Here's how the part is built. I have some questions about the finished solid (model axes, mm). A direction names the side the tool comes from. Coordinates: 2 decimals unless noted, no trailing zeros. Write each loop counter-clockwise with the first axis right and the second up, starting at its lowest first coordinate (ties: lowest second). Pieces come first, ordered by that corner, then holes.
Item 1: I want a section at C-C (z = -1). Please give me the cut outline in (x, y), and give its area (3 significant figures).
Item 2: For faces 1 (the face through (18, 441.047, -4)), 2 (the face through (-6.469, 481, 3)), 3 (the face through (8, 482, 9.934)), 4 (the face through (13.531, 483, 5)), which set-ups out of +Z, -Z, +X, -X, +Y, -Y let a thin tool reach every point of the face, with its end or its side?
Item 3: I want a section at A-A (y = 483). Please give me the cut outline in (x, z).
Item 4: I want a section at D-D (x = -2.5). Please give me the cut outline in (y, z), and give its area (3 significant figures).
Item 5: I'm going to push flat-ended pins straight in: P1, Ø3, axis at x = -3.5, z = 18, coming from the +Y side; P2, Ø2.5, axis at x = -21, z = -3, coming from the +Y side; P3, Ø6, axis at y = 487.55, z = 4.93, coming from the +X side. Where does each tip first touch, or does it pass through?
Item 6: I want a section at B-B (x = -12). Please give me the cut outline in (y, z), and give its area (3 significant figures).
Item 7: If we mould it in two halves opening along Y, with no side actions, what happens to faces 5 (the face through (-8, 469.547, -1)), 6 (the face through (-12, 482, -0.066)), 7 (the face through (-2, 412.547, 29))? For each: pulls with the +Y half, pulls with the -Y half, needs draft (parallel to the pull), parting line crosses it, or undercut.
Item 8: Please list where these lines run through material, in increasing order: line 1 (Y direction, x = -6, z = 4); line 2 (X direction, y = 440.5, z = 3.5); line 3 (X direction, y = 427, z = 23).
from build123d import *

# Parameters (mm, degrees)
SKETCH1_W            = 50
SKETCH1_H            = 40
BOSS_EXTRUDE1_DEPTH  = 10
SKETCH5_W            = 6
SKETCH5_H            = 5
BOSS_EXTRUDE3_DEPTH  = 10
SKETCH6_R            = 2
CUT_EXTRUDE1_DEPTH   = 20
SKETCH8_W            = 10
SKETCH8_H            = 40
CUT_EXTRUDE2_DEPTH   = 25
SKETCH9_W            = 10
SKETCH9_H            = 6
SKETCH9_R            = 1.930897171
BOSS_EXTRUDE4_DEPTH  = 5
SKETCH10_W           = 10
SKETCH10_H           = 5
CUT_EXTRUDE3_DEPTH   = 15
SKETCH11_W           = 5
SKETCH11_H           = 5
BOSS_EXTRUDE5_DEPTH  = 10
SKETCH12_R           = 1.5
CUT_EXTRUDE4_DEPTH   = 10
SKETCH13_W           = 6
SKETCH13_H           = 5
CUT_EXTRUDE5_DEPTH   = 10
SKETCH15_W           = 5
SKETCH15_H           = 5
BOSS_EXTRUDE7_DEPTH  = 10
SKETCH18_W           = 5
SKETCH18_H           = 5
CUT_EXTRUDE7_DEPTH   = 10
SKETCH19_R           = 1.25
CUT_EXTRUDE8_DEPTH   = 43
CUT_EXTRUDE9_DEPTH   = 20
SKETCH21_W           = 16
SKETCH21_H           = 16
CUT_EXTRUDE10_DEPTH  = 30
SKETCH22_W           = 8
SKETCH22_H           = 12
CUT_EXTRUDE11_DEPTH  = 4
SCALE2_SCALE         = 2
CUT_EXTRUDE12_DEPTH  = 30
SKETCH24_W           = 44
SKETCH24_H           = 7
CUT_EXTRUDE13_DEPTH  = 3
SKETCH25_W           = 3
SKETCH25_H           = 8
BOSS_EXTRUDE8_DEPTH  = 8
BOSS_EXTRUDE9_DEPTH  = 2
SKETCH27_W           = 52
SKETCH27_H           = 50
BOSS_EXTRUDE10_DEPTH = 2
BOSS_EXTRUDE11_DEPTH = 2
CUT_EXTRUDE15_DEPTH  = 64


with BuildPart() as part:
    # Sketch1 → Boss-Extrude1 (new body)
    with BuildSketch(Plane(origin=(669.84184187, 0, 0), x_dir=(1, 0, 0), z_dir=(0, 0, 1))):
        with Locations((-671.310344828, 437.637931034)):
            Rectangle(SKETCH1_W, SKETCH1_H)
    boss_extrude1 = extrude(amount=BOSS_EXTRUDE1_DEPTH)

    # Sketch5 → Boss-Extrude3 (add)
    with BuildSketch(Plane(origin=(23.531497042, 0, 0), x_dir=(0, 0, -1), z_dir=(1, 0, 0))):
        with Locations((-5, 442.637931034)):
            Rectangle(SKETCH5_W, SKETCH5_H)
        with Locations((-5, 432.637931034)):
            Rectangle(SKETCH5_W, SKETCH5_H)
    extrude(amount=BOSS_EXTRUDE3_DEPTH)

    # Sketch6 → Cut-Extrude1 (cut)
    with BuildSketch(Plane(origin=(669.84184187, 445.137931034, 0), x_dir=(1, 0, 0), z_dir=(0, 1, 0))):
        with Locations(Location((-641.310344828, -5, 0), (0, 0, 180))):
            Circle(SKETCH6_R)
    extrude(amount=-CUT_EXTRUDE1_DEPTH, mode=Mode.SUBTRACT)

    # Sketch8 → Cut-Extrude2 (cut)
    with BuildSketch(Plane.ZY.offset(26.468502958)):
        with Locations((5, 437.637931034)):
            Rectangle(SKETCH8_W, SKETCH8_H)
    extrude(amount=-CUT_EXTRUDE2_DEPTH, mode=Mode.SUBTRACT)

    # Sketch9 → Boss-Extrude4 (add)
    with BuildSketch(Plane(origin=(0, 435.137931034, 0), x_dir=(1, 0, 0), z_dir=(0, 1, 0))):
        with Locations((28.531497042, -5)):
            Rectangle(SKETCH9_W, SKETCH9_H)
        with Locations(Location((28.531497042, -5, 0), (0, 0, 180))):
            Circle(SKETCH9_R, mode=Mode.SUBTRACT)
    extrude(amount=BOSS_EXTRUDE4_DEPTH)

    # Sketch10 → Cut-Extrude3 (cut)
    with BuildSketch(Plane.XY.offset(8)):
        with Locations((28.531497042, 432.637931034)):
            Rectangle(SKETCH10_W, SKETCH10_H)
        with Locations((28.531497042, 442.637931034)):
            Rectangle(SKETCH10_W, SKETCH10_H)
    extrude(amount=-CUT_EXTRUDE3_DEPTH, mode=Mode.SUBTRACT)

    # Mirror1: Boss-Extrude1 across plane
    add(boss_extrude1.mirror(Plane(origin=(-1.468502958, 0, 0), x_dir=(0, 0, 1), z_dir=(1, 0, 0))))

    # Sketch11 → Boss-Extrude5 (add)
    with BuildSketch(Plane(origin=(0, 457.637931034, 0), x_dir=(1, 0, 0), z_dir=(0, 1, 0))):
        with Locations((-1.468502958, -5)):
            Rectangle(SKETCH11_W, SKETCH11_H)
    extrude(amount=BOSS_EXTRUDE5_DEPTH)

    # Sketch12 → Cut-Extrude4 (cut)
    with BuildSketch(Plane(origin=(1.031497042, 0, 0), x_dir=(0, 0, -1), z_dir=(1, 0, 0))):
        with Locations((-5, 462.637931034)):
            Circle(SKETCH12_R)
    extrude(amount=-CUT_EXTRUDE4_DEPTH, mode=Mode.SUBTRACT)

    # Sketch13 → Cut-Extrude5 (cut)
    with BuildSketch(Plane(origin=(33.531497042, 0, 0), x_dir=(0, 0, -1), z_dir=(1, 0, 0))):
        with Locations((-5, 437.637931034)):
            Rectangle(SKETCH13_W, SKETCH13_H)
    extrude(amount=-CUT_EXTRUDE5_DEPTH, mode=Mode.SUBTRACT)

    # Sketch15 → Boss-Extrude7 (add)
    with BuildSketch(Plane(origin=(0, 457.637931034, 0), x_dir=(1, 0, 0), z_dir=(0, 1, 0))):
        with Locations((-6.468502958, -5)):
            Rectangle(SKETCH15_W, SKETCH15_H)
        with Locations((3.531497042, -5)):
            Rectangle(SKETCH15_W, SKETCH15_H)
    extrude(amount=BOSS_EXTRUDE7_DEPTH)

    # Sketch18 → Cut-Extrude7 (cut)
    with BuildSketch(Plane(origin=(0, 467.637931034, 0), x_dir=(1, 0, 0), z_dir=(0, 1, 0))):
        with Locations((-1.468502958, -5)):
            Rectangle(SKETCH18_W, SKETCH18_H)
    extrude(amount=-CUT_EXTRUDE7_DEPTH, mode=Mode.SUBTRACT)

    # Sketch19 → Cut-Extrude8 (cut)
    with BuildSketch(Plane.ZY.offset(8.968502958)):
        with Locations((5, 462.637931034)):
            Circle(SKETCH19_R)
    extrude(amount=-CUT_EXTRUDE8_DEPTH, mode=Mode.SUBTRACT)

    # Sketch20 → Cut-Extrude9 (cut)
    with BuildSketch(Plane(origin=(6.031497042, 0, 0), x_dir=(0, 0, -1), z_dir=(1, 0, 0))):
        with BuildLine():
            Line((-7.5, 467.637931034), (-7.5, 462.637931034))
            ThreePointArc((-7.5, 462.637931034), (-5, 465.137931034), (-2.5, 462.637931034))
            Line((-2.5, 462.637931034), (-2.5, 467.637931034))
            Line((-2.5, 467.637931034), (-7.5, 467.637931034))
        make_face()
    extrude(amount=-CUT_EXTRUDE9_DEPTH, mode=Mode.SUBTRACT)

    # Sketch21 → Cut-Extrude10 (cut)
    with BuildSketch(Plane.XY.offset(10)):
        with Locations((-1.468502958, 437.637931034)):
            Rectangle(SKETCH21_W, SKETCH21_H)
    extrude(amount=-CUT_EXTRUDE10_DEPTH, mode=Mode.SUBTRACT)

    # Sketch22 → Cut-Extrude11 (cut)
    with BuildSketch(Plane(origin=(0, 0, 0), x_dir=(-1, 0, 0), z_dir=(0, 0, -1))):
        with Locations((1.468502958, 451.637931034)):
            Rectangle(SKETCH22_W, SKETCH22_H)
    extrude(amount=-CUT_EXTRUDE11_DEPTH, mode=Mode.SUBTRACT)


with BuildPart() as part_1:
    # Scale2: scaled about (-1.468502958, 437.728990864, 5.066378231)
    add(part.part.scale(SCALE2_SCALE).moved(Location((1.468502958, -437.728990864, -5.066378231))))

    # Sketch23 → Cut-Extrude12 (cut)
    with BuildSketch(Plane(origin=(0, 0, -5.066378231), x_dir=(-1, 0, 0), z_dir=(0, 0, -1))):
        Polygon((27.468502958, 495.287404552), (27.468502958, 477.546871205), (51.468502958, 477.546871205), (51.468502958, 397.546871205), (-48.531497042, 397.546871205), (-48.531497042, 477.546871205), (-24.531497042, 477.546871205), (-24.531497042, 495.287404552), (-71.530370383, 495.287404552), (-71.530370383, 371.111775085), (85.960671869, 371.111775085), (85.960671869, 495.287404552), align=None)
        Polygon((51.468502958, 477.546871205), (27.468502958, 477.546871205), (27.468502958, 410.546871205), (-24.531497042, 410.546871205), (-24.531497042, 477.546871205), (-48.531497042, 477.546871205), (-48.531497042, 397.546871205), (51.468502958, 397.546871205), align=None)
    extrude(amount=-CUT_EXTRUDE12_DEPTH, mode=Mode.SUBTRACT)

    # Sketch24 → Cut-Extrude13 (cut)
    with BuildSketch(Plane(origin=(0, 0, -5.066378231), x_dir=(-1, 0, 0), z_dir=(0, 0, -1))):
        with Locations((1.468502958, 437.546871205)):
            Rectangle(SKETCH24_W, SKETCH24_H)
    extrude(amount=-CUT_EXTRUDE13_DEPTH, mode=Mode.SUBTRACT)

    # Sketch25 → Boss-Extrude8 (add)
    with BuildSketch(Plane(origin=(0, 0, 2.933621769), x_dir=(-1, 0, 0), z_dir=(0, 0, -1))):
        with Locations((-5.031497042, 473.546871205)):
            Rectangle(SKETCH25_W, SKETCH25_H)
        with Locations((7.968502958, 473.546871205)):
            Rectangle(SKETCH25_W, SKETCH25_H)
    extrude(amount=BOSS_EXTRUDE8_DEPTH)

    # Sketch26 → Boss-Extrude9 (add)
    with BuildSketch(Plane.ZY.offset(27.468502958)):
        Polygon((44.933621769, 410.546871205), (14.933621769, 477.546871205), (14.933621769, 410.546871205), align=None)
    extrude(amount=-BOSS_EXTRUDE9_DEPTH)

    # Sketch27 → Boss-Extrude10 (add)
    with BuildSketch(Plane.XZ.offset(-410.546871205)):
        with Locations((-1.468502958, 19.933621769)):
            Rectangle(SKETCH27_W, SKETCH27_H)
    extrude(amount=-BOSS_EXTRUDE10_DEPTH)

    # Sketch28 → Boss-Extrude11 (add)
    with BuildSketch(Plane(origin=(24.531497042, 0, 0), x_dir=(0, 0, -1), z_dir=(1, 0, 0))):
        Polygon((-14.933621769, 477.546871205), (-44.933621769, 410.546871205), (5.066378231, 410.546871205), align=None)
    extrude(amount=-BOSS_EXTRUDE11_DEPTH)

    # Sketch31 → Cut-Extrude15 (cut)
    with BuildSketch(Plane(origin=(24.531497042, 0, 0), x_dir=(0, 0, -1), z_dir=(1, 0, 0))):
        with BuildLine():
            Line((-42.679814302, 415.580374548), (-51.64215649, 418.145209821))
            Line((-51.64215649, 418.145209821), (-53.81664241, 410.546871205))
            Line((-53.81664241, 410.546871205), (-41.973839944, 407.710599457))
            Line((-41.973839944, 407.710599457), (-39.182920234, 410.546871205))
            ThreePointArc((-39.182920234, 410.546871205), (-41.973839944, 412.339392402), (-42.679814302, 415.580374548))
        make_face()
    extrude(amount=-CUT_EXTRUDE15_DEPTH, mode=Mode.SUBTRACT)


solid = part_1.part
Answer:
1. outline: (-27.47, 410.55) - (24.53, 410.55) - (24.53, 477.55) - (3.53, 477.55) - (3.53, 469.55) - (6.53, 469.55) - (6.53, 453.55) - (14.53, 453.55) - (14.53, 421.55) - (-17.47, 421.55) - (-17.47, 453.55) - (-9.47, 453.55) - (-9.47, 469.55) - (-6.47, 469.55) - (-6.47, 477.55) - (-27.47, 477.55) - close
1. area: 2,120 mm2
2. face 1: -Z
2. face 2: -Z, +Y
2. face 3: +Z, +X, -X, +Y
2. face 4: +Z, -Z, +X, +Y
3. outline: (-16.47, -0.07) - (-6.47, -0.07) - (-6.47, 9.93) - (-16.47, 9.93) - close; (3.53, -0.07) - (13.53, -0.07) - (13.53, 9.93) - (3.53, 9.93) - close
4. outline: (410.55, -5.07) - (421.55, -5.07) - (421.55, 14.93) - (412.55, 14.93) - (412.55, 42.11) arc R4.33 ccw to (410.55, 39.18) - close; (453.55, 2.93) - (477.55, 2.93) - (477.55, 14.93) - (453.55, 14.93) - close
4. area: 560 mm2
5. P1: stops at y = 412.55
5. P2: stops at y = 477.55
5. P3: stops at x = 13.53
6. outline: (410.55, -5.07) - (421.55, -5.07) - (421.55, 14.93) - (412.55, 14.93) - (412.55, 42.11) arc R4.33 ccw to (410.55, 39.18) - close; (453.55, -5.07) - (477.55, -5.07) - (477.55, -0.07) - (487.55, -0.07) arc R5 ccw to (487.55, 9.93) - (477.55, 9.93) - (477.55, 14.93) - (453.55, 14.93) - close; hole circle Ø5 at (487.55, 4.93)
6. area: 872 mm2
7. face 5: undercut
7. face 6: needs draft
7. face 7: pulls with the +Y half
8. line 1: y = 410.55 to 421.55, 453.55 to 477.55
8. line 2: x = -27.47 to -17.47, 14.53 to 24.53
8. line 3: x = -27.47 to -25.47, 22.53 to 24.53
